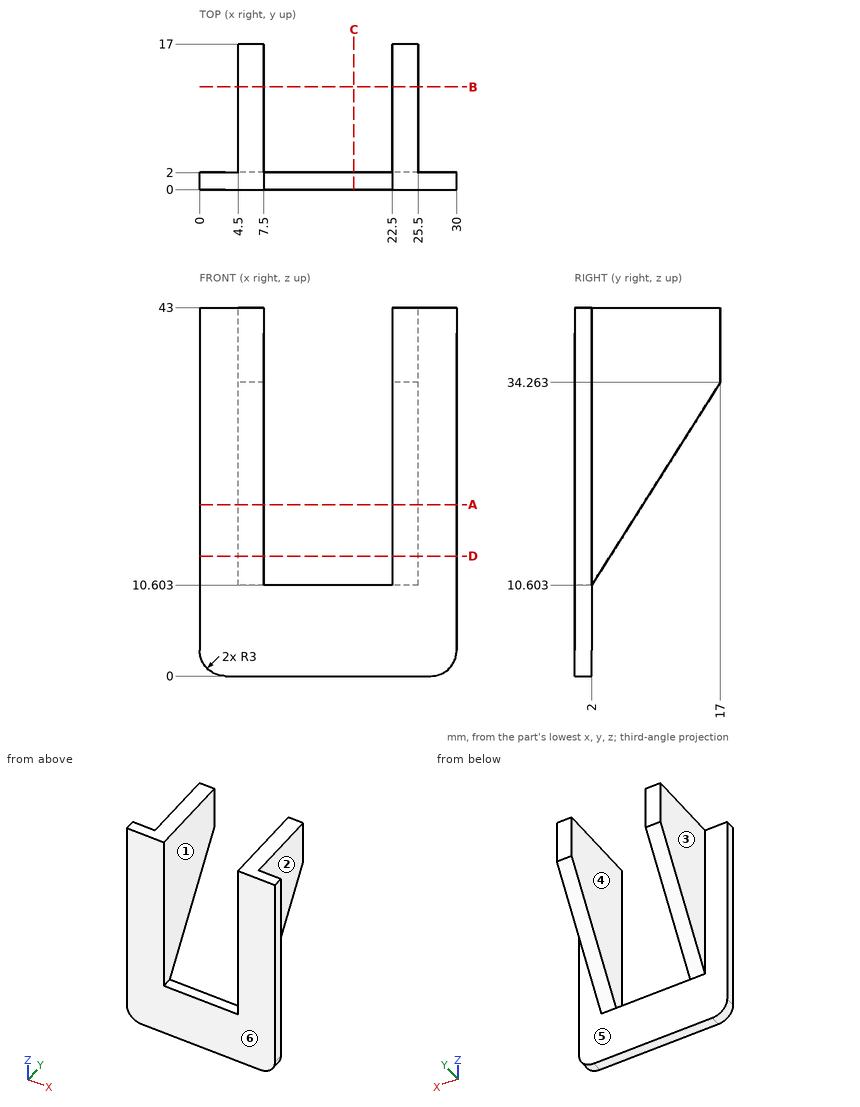
The drawing under review shows one solid part. Ordinate dimensions are in mm from its lowest x, y, z. A direction names the side the tool comes from. Give positions to 0.01 mm unless a question says otherwise; leave off trailing zeros. Order: outer loops, then holes, each group sorted by start corner. A loop starts at its lowest first (then second) coordinate and runs counter-clockwise, first axis right, second up. Notation, with made-up numbers: (79.25, 87.5) - (132.25, 87.5) arc R21 cw to (132.25, 123.5) - close; hole circle Ø6 at (-22, 53). An arc over 180 degrees is marked (long way). Answer as a JSON object with one key per item and string values. Group by question number.
Item 1: Take a section at A-A on z = 20. Give the boundary of the cut face in (x, y).
Item 2: Draft analysis for pull direction X (two halves, no side actions). For the marked faces 1, 2 and 3, state which applies: pulls with the +X half, pulls with the -X half, needs draft (parallel to the pull), parting line crosses it, or undercut.
Item 3: Take a section at C-C on x = 18. Give the boundary of the cut face in (y, z).
Item 4: Machinability: for the marked faces 4, 5 and 6, which of the approach directions +Z, -Z, +X, -X, +Y, -Y give a long, thin tool a straight path to every point of the face, cutting with its end or side? Answer none if there is none.
Item 5: Wall thickness on line 1 along X through (y, z) = (7.75, 22); line 2 along Y through (x, z) = (8.25, 5); line 3 along Y through (x, z) = (5.75, 17.5): over which ranges is each line inside the solid? List them lowest first.
Item 6: Take a section at D-D on z = 14. Give the boundary of the cut face in (x, y).
Item 7: Clearance check with flat-ended pins moving along their axes: pin 1 Ø10 at (x, y) = (15.5, 12.5) entering from -Z; pin 2 Ø7.5 at (y, z) = (7.5, 19) entering from -X; pin 3 Ø1 at (x, y) = (15.5, 1) entering from +Z; pin 4 Ø1.5 at (y, z) = (7.5, 18.5) entering from +X. State where each tip first meets the part, or that it passes through.
Item 8: Take a section at B-B on y = 12. Give the boundary of the cut face in (x, z).
Reported:
{
 "1": {"outline": "(0, 0) - (7.5, 0) - (7.5, 7.96) - (4.5, 7.96) - (4.5, 2) - (0, 2) - close; (22.5, 0) - (30, 0) - (30, 2) - (25.5, 2) - (25.5, 7.96) - (22.5, 7.96) - close"},
 "2": {"face 1": "undercut", "face 2": "pulls with the +X half", "face 3": "pulls with the -X half"},
 "3": {"outline": "(0, 0) - (2, 0) - (2, 10.6) - (0, 10.6) - close"},
 "4": {"face 4": "+Z, +Y, -Y", "face 5": "-Z, +Y", "face 6": "+Z, -Z, +X, -X, -Y"},
 "5": {"line 1": "4.5 to 7.5, 22.5 to 25.5", "line 2": "0 to 2", "line 3": "0 to 6.37"},
 "6": {"outline": "(0, 0) - (7.5, 0) - (7.5, 4.15) - (4.5, 4.15) - (4.5, 2) - (0, 2) - close; (22.5, 0) - (30, 0) - (30, 2) - (25.5, 2) - (25.5, 4.15) - (22.5, 4.15) - close"},
 "7": {"pin 1": "through", "pin 2": "x = 4.5", "pin 3": "z = 10.6", "pin 4": "x = 25.5"},
 "8": {"outline": "(4.5, 26.38) - (7.5, 26.38) - (7.5, 43) - (4.5, 43) - close; (22.5, 26.38) - (25.5, 26.38) - (25.5, 43) - (22.5, 43) - close"}
}
